For this review, take the finished solid that the model builds, in its own axes (mm). Coordinates: 2 decimals unless noted, no trailing zeros. Write each loop counter-clockwise with the first axis right and the second up, starting at its lowest first coordinate (ties: lowest second). Pieces come first, ordered by that corner, then holes.
1) Insertion check: P1, Ø1.5, axis at x = -2.5, z = 9.5, coming from the -Y side; P2, Ø2, axis at x = 0.5, z = 22, coming from the +Y side. Each pin has a flat end and moves straight along its axis. Give the tip position at first contact, or say it passes through.
2) We need section B-B on y = 1. Write out the cut boundary in (x, z), then the cut area to 3 significant figures.
3) We need section C-C on z = 17.5. Write out the cut boundary in (x, y).
4) Mouldability with a two-part tool opening along Z and no side actions: class faces 1 (the face through (0, 0, 36)), 2 (the face through (0, 0, -36)), 3 (the face through (3.434, 1.081, 34.507)), 4 (the face through (3.434, 1.081, -34.507)) as pulls with the +Z half, pulls with the -Z half, needs draft (parallel to the pull), parting line crosses it, or undercut.
5) To check wall thickness, follow line 1 along Y through (x, z) = (-0.25, 15.5); line 2 along Y through (x, z) = (3.5, -19); line 3 along X through (y, z) = (2.5, -21). State the ranges of each line that lie inside material, in increasing order.
6) We need section A-A on x = 1.25. Write out the cut boundary in (y, z).
from build123d import *

# Parameters (mm, degrees)
SKETCH_1_R          = 4
EXTRUDE_1_DEPTH     = 36
CUT_EXTRUDE_START   = 1
SKETCH_2_R          = 4
SKETCH_2_R_2        = 3.6
CUT_EXTRUDE_1_DEPTH = 1


with BuildPart() as part:
    # 草图1 → 凸台-拉伸1 (new, symmetric)
    with BuildSketch(Plane.XY):
        Circle(SKETCH_1_R)
    extrude(amount=EXTRUDE_1_DEPTH, both=True)

    # 草图2 → 切除-拉伸1 (cut)
    with BuildSketch(Plane.XY.offset(34).offset(CUT_EXTRUDE_START)):
        Circle(SKETCH_2_R)
        Circle(SKETCH_2_R_2, mode=Mode.SUBTRACT)
    cut_extrude_1 = extrude(amount=-CUT_EXTRUDE_1_DEPTH, mode=Mode.SUBTRACT)

    # 镜向1: 切除-拉伸1 across plane
    add(cut_extrude_1.mirror(Plane.XY), mode=Mode.SUBTRACT)


solid = part.part
Result:
1. P1: stops at y = -3.6
1. P2: stops at y = 4
2. outline: (-3.87, -36) - (3.87, -36) - (3.87, -35) - (3.46, -35) - (3.46, -34) - (3.87, -34) - (3.87, 34) - (3.46, 34) - (3.46, 35) - (3.87, 35) - (3.87, 36) - (-3.87, 36) - (-3.87, 35) - (-3.46, 35) - (-3.46, 34) - (-3.87, 34) - (-3.87, -34) - (-3.46, -34) - (-3.46, -35) - (-3.87, -35) - close
2. area: 556 mm2
3. outline: circle Ø8 at (0, 0)
4. face 1: pulls with the +Z half
4. face 2: pulls with the -Z half
4. face 3: undercut
4. face 4: undercut
5. line 1: y = -3.99 to 3.99
5. line 2: y = -1.94 to 1.94
5. line 3: x = -3.12 to 3.12
6. outline: (-3.8, -36) - (3.8, -36) - (3.8, -35) - (3.38, -35) - (3.38, -34) - (3.8, -34) - (3.8, 34) - (3.38, 34) - (3.38, 35) - (3.8, 35) - (3.8, 36) - (-3.8, 36) - (-3.8, 35) - (-3.38, 35) - (-3.38, 34) - (-3.8, 34) - (-3.8, -34) - (-3.38, -34) - (-3.38, -35) - (-3.8, -35) - close
